For this review, take the finished solid that the model builds, in its own axes (mm). Coordinates: 2 decimals unless noted, no trailing zeros. Write each loop counter-clockwise with the first axis right and the second up, starting at its lowest first coordinate (ties: lowest second). Pieces come first, ordered by that corner, then holes. Notation, with made-up numbers: (41.25, 79.25) -> (59.25, 79.25) arc R23 ccw to (59.25, 93.25) -> close; hole circle Ø10 at (75, 3). An arc over 180 degrees is marked (long way). One line per item, written item: value. Start each with the question number.
1) Add section B-B (z = 0.9). State how many separate pieces and enclosed holes the cut face has, and give its area (3 significant figures).
2) Add section A-A (x = 58). State the section outline as (y, z) points (3 decimals).
3) For probe 1 along X at (y, z) = (-46, 1.7) (3 decimals); probe 2 along X at (y, z) = (9.5, 1.2); probe 3 along Y at (x, z) = (5, 1.25), list the stretches that pass through material, from the lowest coordinate up. Write a range as from..to.
4) Add section D-D (x = 25.5). State the section outline as (y, z) points (3 decimals).
5) For pin 1 Ø4.5 at (x, y) = (-3.11, -11.59) entering from -Z, flat-tipped, find the tip position at first contact; note if it passes through.
6) Add section C-C (y = -34). State the section outline as (x, z) points (3 decimals).
from build123d import *

# Parameters (mm, degrees)
SKETCH1_R           = 2
SKETCH1_R_2         = 2.5
BOSS_EXTRUDE1_DEPTH = 3.175
FILLET1_R           = 5
CHAMFER1_SIZE       = 2.2


with BuildPart() as part:
    # Sketch1 → Boss-Extrude1 (new body)
    with BuildSketch(Plane.XY):
        with BuildLine():
            Line((34.261326859, -49.751843123), (-10.721932331, -13.1924284))
            ThreePointArc((-10.721932331, -13.1924284), (-13.1924284, 10.721932331), (10.721932331, 13.1924284))
            Line((10.721932331, 13.1924284), (55.705191521, -23.366986323))
            ThreePointArc((55.705191521, -23.366986323), (63.295065064, -33.021160716), (66, -45))
            Line((66, -45), (66, -52.5))
            Line((66, -52.5), (42, -52.5))
            ThreePointArc((42, -52.5), (37.893924373, -51.792566974), (34.261326859, -49.751843123))
        make_face()
        with Locations((-8.485281374, 8.485281374)):
            Circle(SKETCH1_R, mode=Mode.SUBTRACT)
        with Locations((3.105828541, 11.591109915)):
            Circle(SKETCH1_R, mode=Mode.SUBTRACT)
        with Locations((11.591109915, 3.105828541)):
            Circle(SKETCH1_R, mode=Mode.SUBTRACT)
        with Locations((8.485281374, -8.485281374)):
            Circle(SKETCH1_R, mode=Mode.SUBTRACT)
        with Locations((42, -45)):
            Circle(SKETCH1_R_2, mode=Mode.SUBTRACT)
        with Locations((58, -45)):
            Circle(SKETCH1_R_2, mode=Mode.SUBTRACT)
        with Locations((-3.105828541, -11.591109915)):
            Circle(SKETCH1_R, mode=Mode.SUBTRACT)
        with Locations((-11.591109915, -3.105828541)):
            Circle(SKETCH1_R, mode=Mode.SUBTRACT)
    extrude(amount=BOSS_EXTRUDE1_DEPTH)

    # Fillet1
    fillet1_edges = [part.edges().sort_by_distance(p)[0] for p in [
        (66, -52.5, 1.5875),
    ]]
    fillet(fillet1_edges, radius=FILLET1_R)

    # Chamfer1
    chamfer1_edges = [part.edges().sort_by_distance(p)[0] for p in [
        (-10.485281374, 8.485281374, 0),
        (1.105828541, 11.591109915, 0),
        (9.591109915, 3.105828541, 0),
        (6.485281374, -8.485281374, 0),
        (-5.105828541, -11.591109915, 0),
        (-13.591109915, -3.105828541, 0),
    ]]
    chamfer(chamfer1_edges, length=CHAMFER1_SIZE)


solid = part.part
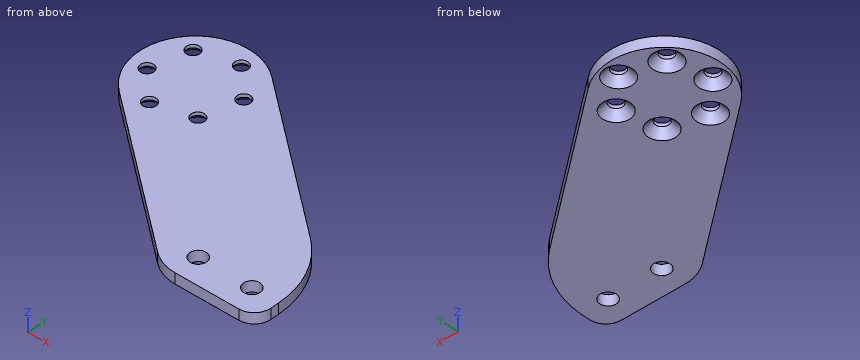
Numbers:
1. separate pieces: 1
1. enclosed holes: 8
1. area: 2,740 mm²
2. outline: (-52.5, 0) -> (-47.5, 0) -> (-47.5, 3.175) -> (-52.5, 3.175) -> close; (-42.5, 0) -> (-25.454, 0) -> (-25.454, 3.175) -> (-42.5, 3.175) -> close
3. probe 1: 29.645..39.709, 44.291..55.709, 60.291..66
3. probe 2: -14.1..-11.31, -5.66..0.95, 5.26..15.27
3. probe 3: -25.97..9.33, 13.85..16.25
4. outline: (-42.631, 0) -> (1.182, 0) -> (1.182, 3.175) -> (-42.631, 3.175) -> close
5. pin 1: z = 1.95
6. outline: (14.88, 0) -> (63.738, 0) -> (63.738, 3.175) -> (14.88, 3.175) -> close
